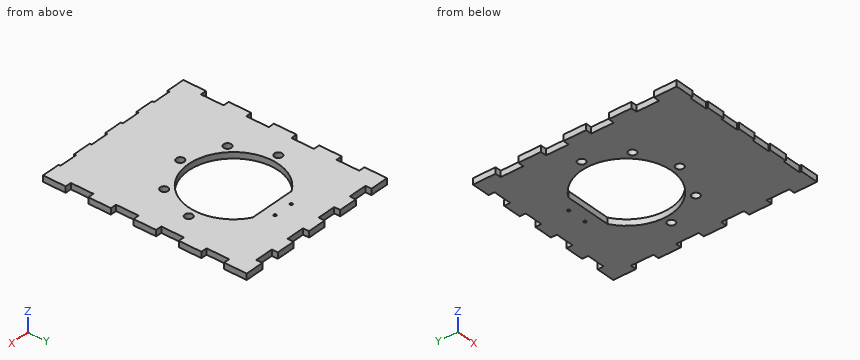
from build123d import *

# Parameters (mm, degrees)
SKETCH1_W           = 137.16
SKETCH1_H           = 167.64
BOSS_EXTRUDE1_DEPTH = 4.9609375
CUT_EXTRUDE1_DEPTH  = 5.9609375
SKETCH4_R           = 3.1877
CUT_EXTRUDE2_DEPTH  = 5.9609375
SKETCH6_W           = 4.9634902
SKETCH6_H           = 18.6182
SKETCH6_W_2         = 15.24
SKETCH6_H_2         = 4.9634902
SKETCH6_H_3         = 1.5875
CUT_EXTRUDE5_DEPTH  = 5.9609375
SKETCH7_OUTSIDE_W   = 182.492
SKETCH7_OUTSIDE_H   = 212.972
SKETCH7_OUTSIDE_R   = 1.1049
CUT_EXTRUDE6_DEPTH  = 5.9609375


with BuildPart() as part:
    # Sketch1 → Boss-Extrude1 (new body)
    with BuildSketch(Plane.XY):
        with Locations((0, -15.24)):
            Rectangle(SKETCH1_W, SKETCH1_H)
    extrude(amount=BOSS_EXTRUDE1_DEPTH)

    # Sketch2 → Cut-Extrude1 (cut, through all)
    with BuildSketch(Plane.XY.offset(4.9609375)):
        with BuildLine():
            Line((-19.05, 31.75), (19.05, 31.75))
            ThreePointArc((19.05, 31.75), (0, -37.026544532), (-19.05, 31.75))
        make_face()
    extrude(amount=-CUT_EXTRUDE1_DEPTH, mode=Mode.SUBTRACT)

    # Sketch4 → Cut-Extrude2 (cut, through all)
    with BuildSketch(Plane.XY.offset(4.9609375)):
        with Locations((-43.815, 0)):
            Circle(SKETCH4_R)
        with Locations((-30.981883618, -30.981883618)):
            Circle(SKETCH4_R)
        with Locations((0, -43.815)):
            Circle(SKETCH4_R)
        with Locations((30.981883618, -30.981883618)):
            Circle(SKETCH4_R)
        with Locations((43.815, 0)):
            Circle(SKETCH4_R)
    extrude(amount=-CUT_EXTRUDE2_DEPTH, mode=Mode.SUBTRACT)

    # Sketch6 → Cut-Extrude5 (cut, through all)
    with BuildSketch(Plane.XY.offset(4.9609375)):
        with Locations((-66.0982549, 3.4163)):
            Rectangle(SKETCH6_W, SKETCH6_H)
        with Locations((-66.0982549, 40.6527)):
            Rectangle(SKETCH6_W, SKETCH6_H)
        with Locations((-66.0982549, -33.8201)):
            Rectangle(SKETCH6_W, SKETCH6_H)
        with Locations((-66.0982549, -71.0565)):
            Rectangle(SKETCH6_W, SKETCH6_H)
        with Locations((66.0982549, 3.40868)):
            Rectangle(SKETCH6_W, SKETCH6_H)
        with Locations((66.0982549, 40.64508)):
            Rectangle(SKETCH6_W, SKETCH6_H)
        with Locations((66.0982549, -33.82772)):
            Rectangle(SKETCH6_W, SKETCH6_H)
        with Locations((66.0982549, -71.06412)):
            Rectangle(SKETCH6_W, SKETCH6_H)
        with Locations((-15.24, 66.0982549)):
            Rectangle(SKETCH6_W_2, SKETCH6_H_2)
        with Locations((-45.72, 66.0982549)):
            Rectangle(SKETCH6_W_2, SKETCH6_H_2)
        with Locations((15.24, 66.0982549)):
            Rectangle(SKETCH6_W_2, SKETCH6_H_2)
        with Locations((45.72, 66.0982549)):
            Rectangle(SKETCH6_W_2, SKETCH6_H_2)
        with Locations((-15.24, -98.26625)):
            Rectangle(SKETCH6_W_2, SKETCH6_H_3)
        with Locations((-45.72, -98.26625)):
            Rectangle(SKETCH6_W_2, SKETCH6_H_3)
        with Locations((15.24, -98.26625)):
            Rectangle(SKETCH6_W_2, SKETCH6_H_3)
        with Locations((45.72, -98.26625)):
            Rectangle(SKETCH6_W_2, SKETCH6_H_3)
    extrude(amount=-CUT_EXTRUDE5_DEPTH, mode=Mode.SUBTRACT)

    # Sketch7 outside → Cut-Extrude6 (cut, through all)
    with BuildSketch(Plane.XY.offset(4.9609375)):
        with Locations((0, -15.24)):
            Rectangle(SKETCH7_OUTSIDE_W, SKETCH7_OUTSIDE_H)
        Polygon((-63.6165098, 49.9618), (-63.6165098, 31.3436), (-68.58, 31.3436), (-68.58, 12.7254), (-63.6165098, 12.7254), (-63.6165098, -5.8928), (-68.58, -5.8928), (-68.58, -24.511), (-63.6165098, -24.511), (-63.6165098, -43.1292), (-68.58, -43.1292), (-68.58, -61.7474), (-63.6165098, -61.7474), (-63.6165098, -80.3656), (-68.58, -80.3656), (-68.58, -99.06), (-53.34, -99.06), (-53.34, -97.4725), (-38.1, -97.4725), (-38.1, -99.06), (-22.86, -99.06), (-22.86, -97.4725), (-7.62, -97.4725), (-7.62, -99.06), (7.62, -99.06), (7.62, -97.4725), (22.86, -97.4725), (22.86, -99.06), (38.1, -99.06), (38.1, -97.4725), (53.34, -97.4725), (53.34, -99.06), (68.58, -99.06), (68.58, -80.37322), (63.6165098, -80.37322), (63.6165098, -61.75502), (68.58, -61.75502), (68.58, -43.13682), (63.6165098, -43.13682), (63.6165098, -24.51862), (68.58, -24.51862), (68.58, -5.90042), (63.6165098, -5.90042), (63.6165098, 12.71778), (68.58, 12.71778), (68.58, 31.33598), (63.6165098, 31.33598), (63.6165098, 49.95418), (68.58, 49.95418), (68.58, 68.58), (53.34, 68.58), (53.34, 63.6165098), (38.1, 63.6165098), (38.1, 68.58), (22.86, 68.58), (22.86, 63.6165098), (7.62, 63.6165098), (7.62, 68.58), (-7.62, 68.58), (-7.62, 63.6165098), (-22.86, 63.6165098), (-22.86, 68.58), (-38.1, 68.58), (-38.1, 63.6165098), (-53.34, 63.6165098), (-53.34, 68.58), (-68.58, 68.58), (-68.58, 49.9618), align=None, mode=Mode.SUBTRACT)
        with Locations((-7.9375, 40.87749)):
            Circle(SKETCH7_OUTSIDE_R)
        with Locations((7.9375, 40.87749)):
            Circle(SKETCH7_OUTSIDE_R)
    extrude(amount=-CUT_EXTRUDE6_DEPTH, mode=Mode.SUBTRACT)


solid = part.part
CAD build for the part. Positions are in the model's coordinates, mm. Coordinates: 2 decimals unless noted, no trailing zeros. Write each loop counter-clockwise with the first axis right and the second up, starting at its lowest first coordinate (ties: lowest second). Pieces come first, ordered by that corner, then holes. Notation, with made-up numbers: (-12, 67) - (-3, 67) arc R22 cw to (-3, 92) - close; hole circle Ø6 at (69.5, 12.25). An arc over 180 degrees is marked (long way). Use a Markdown table: item, result. Add a question column.
Item 1: Band-saw the part on A-A, the plane x = 0. Give the cut face in (y, z), and give its area (3 significant figures).
Item 2: Band-saw the part on B-B, the plane y = 0. Give the cut face in (x, z), and give its area (3 significant figures).
Item 3: Drill centre lines: L1, parallel to Y at x = 0, z = 3.85; L2, parallel to Y at x = 2, z = 1.1; L3, parallel to X at y = 25, z = 2.75. Where is each one in solid material? Low to high. Write a range as from..to.
Item 4: Band-saw the part on C-C, the plane z = 1.8. Give the number of separate pieces and of enclosed holes in the cut face, and give its area (3 significant figures).
Numbers:
| question | item | result |
|---|---|---|
| 1 | outline | (-99.06, 0) - (-47, 0) - (-47, 4.96) - (-99.06, 4.96) - close; (-40.63, 0) - (-37.03, 0) - (-37.03, 4.96) - (-40.63, 4.96) - close; (31.75, 0) - (68.58, 0) - (68.58, 4.96) - (31.75, 4.96) - close |
| 1 | area | 459 mm2 |
| 2 | outline | (-63.62, 0) - (-47, 0) - (-47, 4.96) - (-63.62, 4.96) - close; (-40.63, 0) - (-37.03, 0) - (-37.03, 4.96) - (-40.63, 4.96) - close; (37.03, 0) - (40.63, 0) - (40.63, 4.96) - (37.03, 4.96) - close; (47, 0) - (63.62, 0) - (63.62, 4.96) - (47, 4.96) - close |
| 2 | area | 201 mm2 |
| 3 | L1 | -99.06..-47, -40.63..-37.03, 31.75..68.58 |
| 3 | L2 | -99.06..-46.3, -41.33..-36.97, 31.75..68.58 |
| 3 | L3 | -68.58..-27.31, 27.31..68.58 |
| 4 | separate pieces | 1 |
| 4 | enclosed holes | 8 |
| 4 | area | 17,500 mm2 |
